For this review, take the finished solid that the model builds, in its own axes (mm). A direction names the side the tool comes from. Coordinates: 2 decimals unless noted, no trailing zeros. Order: outer loops, then holes, each group sorted by start corner. A loop starts at its lowest first (then second) coordinate and runs counter-clockwise, first axis right, second up. Notation, with made-up numbers: (28, -14.75) -> (44, -14.75) arc R29 cw to (44, 22.25) -> close; hole circle Ø6 at (88, 41.25). An arc over 180 degrees is marked (long way). Return JSON: item names as keys, results as strings. Group by question number.
Item 1: Machinability: for faces 4 (the cylindrical face through (172.55, -7.509, -23.846)), 5 (the cylindrical face through (437.32, -299.32, -20.16)), 6 (the cylindrical face through (573.25, -7.509, -23.846)), which of the approach directions +Z, -Z, +X, -X, +Y, -Y give a long, thin tool a straight path to every point of the face, cutting with its end or side? Answer none if there is none.
Item 2: Take a section at A-A (z = -43.5). Write out the cut boundary in (x, y).
Item 3: Take a section at D-D (z = 247.5). Write out the cut boundary in (x, y), then the cut area to 3 significant figures.
Item 4: For line 1 along X through (y, z) = (-195, 227.5); line 2 along Z through (x, y) = (405, 2); line 3 along Z through (x, y) = (643.5, -1), list the stretches that pass through material, from the lowest coordinate up.
Item 5: Take a section at B-B (y = 54). Write out the cut boundary in (x, z), then the cut area to 3 significant figures.
Item 6: Take a section at C-C (x = 147). Write out the cut boundary in (y, z), then the cut area to 3 significant figures.
Item 7: Insertion check: pin 1 (3 mm diameter, centred on y = 171.5, z = 173.5, fed in from +X); pin 2 (6 mm diameter, centred on y = 189, z = 233.5, fed in from -X); pin 3 (12 mm diameter, centred on x = 355, y = 142.5, fed in from -Z). Each pin has a flat end and moves straight along its axis. Give the tip position at first contact, or say it passes through.
Item 8: Draft analysis for pull direction X (two halves, no side actions). For faces 1 (the cylindrical face through (923.25, -7.509, -23.846)), 2 (the flat face through (450, -63, 3)), 3 (the flat face through (350, -62, -6)), state which applies: +X half, -X half, draft (parallel to the pull), parting line (faces both ways), or undercut.
Autodesk Inventor part; units mm, degrees
ref_plane "YZ Plane" through (0, 0, 0) normal (1, 0, 0) x (0, 1, 0)
ref_plane "XZ Plane" through (0, 0, 0) normal (0, 1, 0) x (-1, 0, 0)
ref_plane "XY Plane" through (0, 0, 0) normal (0, 0, 1) x (1, 0, 0)
sketch "Sketch1" plane through (0, 0, 0) normal (0, 1, 0) x (-1, 0, 0)
  line L0 (0, 0) -> (-400, 0) construction
  line L1 (-400, 0) -> (-750, 0)
  line L2 (-750, 0) -> (-1050, 0)
  line L3 (-400, 0) -> (-400, -300) construction
  line L4 (-400, -300) -> (-375, -300) construction
  line L5 (-375, -300) -> (-425, -300)
  line L6 (-425, -300) -> (-425, 0)
  line L7 (-425, 0) -> (-375, 0)
  line L8 (-375, 0) -> (-375, -300)
  line L9 (0, 0) -> (-1050, 0)
  line L10 (-1050, 0) -> (-1050, -25)
  line L11 (-1050, -25) -> (0, -25)
  line L12 (0, -25) -> (0, 0)
  arc A0 (0, -25) -> (25, 0) centre (0, 0) ccw
  line L13 (0, 0) -> (25, 0) construction
  line L14 (-750, 0) -> (-750, -150) construction
  line L15 (-750, -150) -> (-725, -150) construction
  line L16 (-725, -150) -> (-775, -150)
  line L17 (-775, -150) -> (-775, 0)
  line L18 (-775, 0) -> (-725, 0)
  line L19 (-725, 0) -> (-725, -150)
  arc A1 (-1075, 0) -> (-1050, -25) centre (-1050, 0) ccw
  line L20 (-1050, 0) -> (-1075, 0)
  line L21 (25, 0) -> (0, 0)
  point P0 (-775, -25)
  point P1 (-725, -25)
  point P2 (-425, -25)
  point P3 (-375, -25)
  dimension "d0" = 400
  dimension "d1" = 350
  dimension "d2" = 300
  dimension "d3" = 300
  dimension "d4" = 25
  dimension "d5" = 50
  dimension "d6" = 1050
  dimension "d7" = 25
  dimension "d8" = 150
  dimension "d9" = 25
  dimension "d10" = 50
revolve "Revolution1" add sketch "Sketch1" angle 360 about axis through (0, 0, 0) along (1, 0, 0)
sketch "Sketch2" plane through (375, 0, 0) normal (-1, 0, 0) x (0, 0, 1)
  circle A0 centre (0, 0) radius 300
  line L0 (0, 300) -> (0, 290)
  line L1 (0, 290) -> (25.5833, 307.4702)
  point P0 (14.1547, 299.6659)
  dimension "d12" = 10
extrude "Extrusion1" cut sketch "Sketch2" against normal blind 284.25 contours A0 L1 L0 picked at (7.8644, 296.5058)
sketch "Sketch3" plane through (775, 0, 0) normal (1, 0, 0) x (0, 0, -1)
  circle A0 centre (0, 0) radius 150
  line L0 (0, 150) -> (0, 140)
  line L1 (0, 140) -> (62.4254, 176.0413)
  point P0 (15.8635, 149.1588)
  dimension "d15" = 10
  dimension "d16" = 60
extrude "Extrusion2" cut sketch "Sketch3" against normal blind 139 contours A0 L1 L0 picked at (8.8167, 146.2616)
sketch "Sketch4" plane through (375, 0, 0) normal (-1, 0, 0) x (0, -0.0235977, 0.9997215)
  line L0 (7.0793, 299.9165) -> (-6.8433, 289.9192)
  line L1 (-6.8433, 289.9192) -> (-7.0793, 299.9165)
  arc A0 (-7.0793, 299.9165) -> (7.0793, 299.9165) centre (0, 0) ccw
  circle A1 centre (0, 0) radius 25
sketch "Sketch5" plane through (425, 0, 0) normal (1, 0, 0) x (0, 0.0235977, -0.9997215)
  line L0 (6.8433, 289.9192) -> (-7.0793, 299.9165)
  arc A0 (-7.0793, 299.9165) -> (7.0793, 299.9165) centre (0, 0) ccw
  line L1 (7.0793, 299.9165) -> (6.8433, 289.9192)
  circle A1 centre (0, 0) radius 25
sketch "Sketch6" plane through (725, 140, 0) normal (-1, 0, 0) x (0, 0, 1)
  line L0 (0, 0) -> (-15.8635, 9.1588)
  arc A0 (-15.8635, 9.1588) -> (0, 10) centre (0, -140) ccw
  line L1 (0, 10) -> (0, 0)
  circle A1 centre (0, -140) radius 25
sketch "Sketch7" plane through (775, 140, 0) normal (1, 0, 0) x (0, 0, -1)
  circle A0 centre (0, -140) radius 25
  line L0 (15.8635, 9.1588) -> (0, 0)
  line L1 (0, 0) -> (0, 10)
  arc A1 (0, 10) -> (15.8635, 9.1588) centre (0, -140) ccw
extrude "Extrusion3" add sketch "Sketch6" along normal blind 25 contours L1 A0 L0 | A1
extrude "Extrusion4" add sketch "Sketch7" along normal blind 25
extrude "Extrusion5" add sketch "Sketch5" along normal blind 25
extrude "Extrusion6" add sketch "Sketch4" along normal blind 25
properties part number "shaft_model_10cm" material "Steel"
Findings below:
{
 "1": {"face 4": "-X", "face 5": "+X, -X", "face 6": "none"},
 "2": {"outline": "(350, -296.83) -> (425, -296.83) -> (450, -296.83) -> (450, 296.83) -> (375, 296.83) -> (350, 296.83) -> close; (700, -143.55) -> (775, -143.55) -> (800, -143.55) -> (800, 143.55) -> (725, 143.55) -> (700, 143.55) -> close"},
 "3": {"outline": "(350, -169.54) -> (425, -169.54) -> (450, -169.54) -> (450, 169.54) -> (375, 169.54) -> (350, 169.54) -> close", "area": "33,900 mm2"},
 "4": {"line 1": "x = 350 to 450", "line 2": "z = -299.99 to 299.99", "line 3": "z = -24.98 to 24.98"},
 "5": {"outline": "(350, -295.1) -> (375, -295.1) -> (450, -295.1) -> (450, 295.1) -> (425, 295.1) -> (350, 295.1) -> close; (700, -139.94) -> (725, -139.94) -> (800, -139.94) -> (800, 139.94) -> (775, 139.94) -> (700, 139.94) -> close", "area": "87,000 mm2"},
 "6": {"outline": "circle Ø50 at (0, 0)", "area": "1,960 mm2"},
 "7": {"pin 1": "stops at x = 450", "pin 2": "stops at x = 350", "pin 3": "stops at z = -267.15"},
 "8": {"face 1": "draft", "face 2": "undercut", "face 3": "-X half"}
}
